Input: dimensioned drawing with shaded views. Units: mm. Origin: part minimum x, y, z. Give positions to 0.01 mm unless a question says otherwise; leave off trailing zeros. Answer in a Markdown table with one row per item. Add a question column.
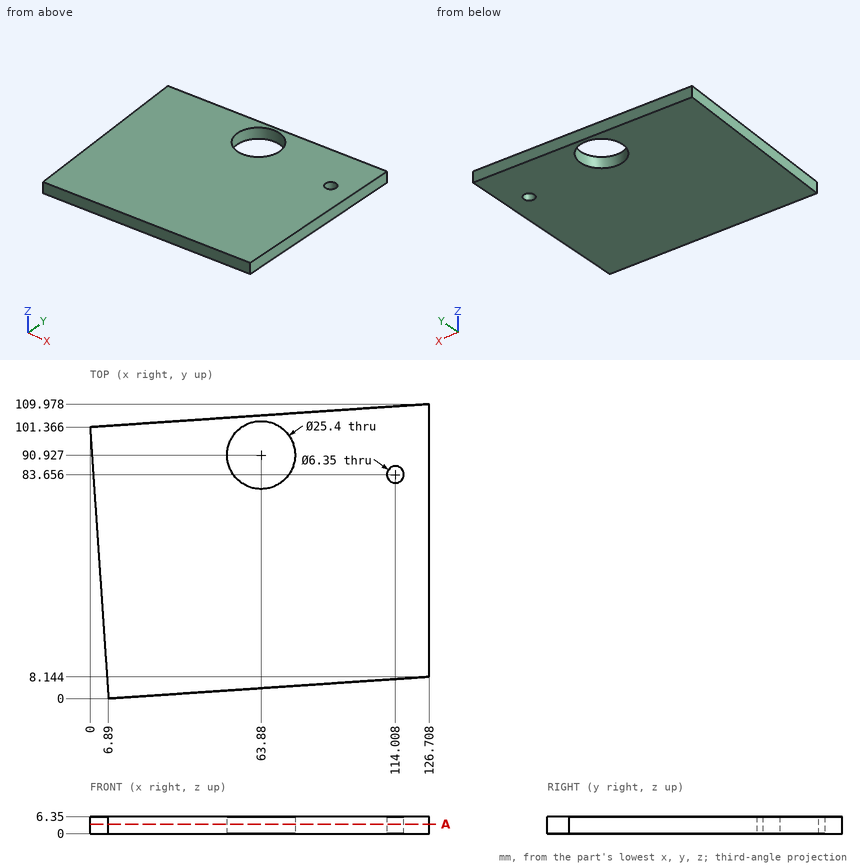
Q1. Line query: probe 1 along X at (y, z) = (82, 2.75) (1 decimal); probe 2 along Y at (x, z) = (64, 4) (1 decimal); probe 3 along X at (y, z) = (17.5, 1). Output: solid intervals per line, ascending. Write a range as from..to.
Q2. Section A-A on z = 3.5. Count the separate pieces of the cut face and the enclosed holes in it, and give its area (3 significant figures).
Q3. Contact query for flat-ended pins moving along their axis: pin 1 Ø1.5 at (y, z) = (88, 1) entering from -X; pin 2 Ø10 at (x, y) = (15.5, 46) entering from -Z; pin 3 Ø1 at (x, z) = (99, 2) entering from +Y. Output: stop coordinate, or through.
Checks:
| question | item | result |
|---|---|---|
| 1 | probe 1 | 1.3..54.8, 72.9..111.3, 116.7..126.7 |
| 1 | probe 2 | 3.9..78.2, 103.6..105.7 |
| 1 | probe 3 | 5.7..126.71 |
| 2 | separate pieces | 1 |
| 2 | enclosed holes | 2 |
| 2 | area | 12,000 mm^2 |
| 3 | pin 1 | x = 0.86 |
| 3 | pin 2 | z = 0 |
| 3 | pin 3 | y = 108.13 |
